Source: CAD feature listing. Evaluate the final solid. Frame: model axes, mm. Coordinates: 2 decimals unless noted, no trailing zeros. Loops run counter-clockwise (first coordinate to the right, second up) from the corner with the lowest first, then second, coordinate; pieces in that order, holes last. Notation, with made-up numbers: (70, 5) -> (105, 5) arc R19 ccw to (105, 27) -> close; hole circle Ø8 at (44.5, 63). An arc over 180 degrees is marked (long way). Answer as a JSON object with one key per item and string values. Group by question number.
from build123d import *

# Parameters (mm, degrees)
F0_W         = 150
F0_H         = 73.4827055006
F0_R         = 15.3666463422
F0_R_2       = 9.9309311283
F1_DEPTH     = 76.962
F2_T1_DEPTH  = 139.84
F2_T3_DEPTH  = 63.3227055006
F2_T5_DEPTH  = 157.62
F2_T7_DEPTH  = 81.1027055006
F2_T9_DEPTH  = 84.582
F2_S13_W     = 5.08
F2_S13_H     = 5.08
F2_T14_DEPTH = 5.08
F2_S19_W     = 5.08
F2_S19_H     = 5.08
F2_T20_DEPTH = 5.08
F2_S25_W     = 5.08
F2_S25_H     = 5.08
F2_T26_DEPTH = 5.08


# Not quite as in the source:
# - a fillet or chamfer that OpenCascade refuses, or shapes differently, is made with other operations: its cross-section is extruded or revolved along the edge and cut away or added


with BuildPart() as f1:
    # F0 (on Top) → F1 (new body)
    with BuildSketch(Plane.XY):
        with Locations((19.2005559802, -34.1252638027)):
            Rectangle(F0_W, F0_H)
        with Locations((51.502276212, -42.9059304297)):
            Circle(F0_R, mode=Mode.SUBTRACT)
        with Locations((-28.6887511611, -14.8067288101)):
            Circle(F0_R_2, mode=Mode.SUBTRACT)
    extrude(amount=F1_DEPTH)

    # F2: fillet of radius 5.08 on 9 edges, made by hand

    # F2_s2 → F2_t1 (cut)
    with BuildSketch(Plane.YZ.offset(-50.7194440198)):
        with BuildLine():
            ThreePointArc((-70.866616553, 71.882), (-69.3787190014, 75.4741024484), (-65.786616553, 76.962))
            Line((-65.786616553, 76.962), (-70.866616553, 76.962))
            Line((-70.866616553, 76.962), (-70.866616553, 71.882))
        make_face()
    extrude(amount=F2_T1_DEPTH, mode=Mode.SUBTRACT)

    # F2_s4 → F2_t3 (cut)
    with BuildSketch(Plane.XZ.offset(2.4639110524)):
        with BuildLine():
            ThreePointArc((94.2005559802, 71.882), (92.7126584286, 75.4741024484), (89.1205559802, 76.962))
            Line((89.1205559802, 76.962), (94.2005559802, 76.962))
            Line((94.2005559802, 76.962), (94.2005559802, 71.882))
        make_face()
    extrude(amount=F2_T3_DEPTH, mode=Mode.SUBTRACT)

    # F2_s6 → F2_t5 (cut)
    with BuildSketch(Plane.YZ.offset(-68.4994440198)):
        with BuildLine():
            ThreePointArc((2.6160889476, 71.882), (1.128191396, 75.4741024484), (-2.4639110524, 76.962))
            Line((-2.4639110524, 76.962), (2.6160889476, 76.962))
            Line((2.6160889476, 76.962), (2.6160889476, 71.882))
        make_face()
    extrude(amount=F2_T5_DEPTH, mode=Mode.SUBTRACT)

    # F2_s8 → F2_t7 (cut)
    with BuildSketch(Plane.XZ.offset(-15.3160889476)):
        with BuildLine():
            ThreePointArc((-55.7994440198, 71.882), (-54.3115464682, 75.4741024484), (-50.7194440198, 76.962))
            Line((-50.7194440198, 76.962), (-55.7994440198, 76.962))
            Line((-55.7994440198, 76.962), (-55.7994440198, 71.882))
        make_face()
    extrude(amount=F2_T7_DEPTH, mode=Mode.SUBTRACT)

    # F2_s10 → F2_t9 (cut)
    with BuildSketch(Plane.XY.offset(-12.7)):
        with BuildLine():
            ThreePointArc((89.1205559802, -70.866616553), (92.7126584286, -69.3787190014), (94.2005559802, -65.786616553))
            Line((94.2005559802, -65.786616553), (94.2005559802, -70.866616553))
            Line((94.2005559802, -70.866616553), (89.1205559802, -70.866616553))
        make_face()
        with BuildLine():
            ThreePointArc((89.1205559802, 2.6160889476), (92.7126584286, 1.128191396), (94.2005559802, -2.4639110524))
            Line((94.2005559802, -2.4639110524), (94.2005559802, 2.6160889476))
            Line((94.2005559802, 2.6160889476), (89.1205559802, 2.6160889476))
        make_face()
        with BuildLine():
            ThreePointArc((-55.7994440198, -65.786616553), (-54.3115464682, -69.3787190014), (-50.7194440198, -70.866616553))
            Line((-50.7194440198, -70.866616553), (-55.7994440198, -70.866616553))
            Line((-55.7994440198, -70.866616553), (-55.7994440198, -65.786616553))
        make_face()
    extrude(amount=F2_T9_DEPTH, mode=Mode.SUBTRACT)


with BuildPart() as f2_tool12:
    # F2_s13 → F2_t14 (new body)
    with BuildSketch(Plane.YZ.offset(-50.7194440198)):
        with Locations((-68.326616553, 74.422)):
            Rectangle(F2_S13_W, F2_S13_H)
    extrude(amount=-F2_T14_DEPTH)

    # F2_s15 → F2_t16 (revolve, cut)
    with BuildSketch(Plane(origin=(-50.7194440198, -65.786616553, 71.882), x_dir=(0, 0.7071067812, -0.7071067812), z_dir=(0, 0.7071067812, 0.7071067812))):
        with BuildLine():
            ThreePointArc((0, -5.08), (5.08, 0), (0, 5.08))
            Line((0, 5.08), (0, -5.08))
        make_face()
    revolve(axis=Axis((-50.7194440198, -65.786616553, 71.882), (-1, 0, 0)), mode=Mode.SUBTRACT)


with BuildPart() as f1_1:
    add(f1.part)

    # F2_t11: cut F2_tool12
    add(f2_tool12.part, mode=Mode.SUBTRACT)


with BuildPart() as f2_tool18:
    # F2_s19 → F2_t20 (new body)
    with BuildSketch(Plane.XZ.offset(65.786616553)):
        with Locations((91.6605559802, 74.422)):
            Rectangle(F2_S19_W, F2_S19_H)
    extrude(amount=F2_T20_DEPTH)

    # F2_s21 → F2_t22 (revolve, cut)
    with BuildSketch(Plane(origin=(89.1205559802, -65.786616553, 71.882), x_dir=(-0.7071067812, 0, -0.7071067812), z_dir=(-0.7071067812, 0, 0.7071067812))):
        with BuildLine():
            ThreePointArc((0, -5.08), (5.08, 0), (0, 5.08))
            Line((0, 5.08), (0, -5.08))
        make_face()
    revolve(axis=Axis((89.1205559802, -65.786616553, 71.882), (0, -1, 0)), mode=Mode.SUBTRACT)


with BuildPart() as f1_2:
    add(f1_1.part)

    # F2_t17: cut F2_tool18
    add(f2_tool18.part, mode=Mode.SUBTRACT)


with BuildPart() as f2_tool24:
    # F2_s25 → F2_t26 (new body)
    with BuildSketch(Plane.XZ.offset(2.4639110524)):
        with Locations((91.6605559802, 74.422)):
            Rectangle(F2_S25_W, F2_S25_H)
    extrude(amount=-F2_T26_DEPTH)

    # F2_s27 → F2_t28 (revolve, cut)
    with BuildSketch(Plane(origin=(89.1205559802, -2.4639110524, 71.882), x_dir=(-0.7071067812, 0, -0.7071067812), z_dir=(0.7071067812, 0, -0.7071067812))):
        with BuildLine():
            ThreePointArc((0, -5.08), (5.08, 0), (0, 5.08))
            Line((0, 5.08), (0, -5.08))
        make_face()
    revolve(axis=Axis((89.1205559802, -2.4639110524, 71.882), (0, 1, 0)), mode=Mode.SUBTRACT)


with BuildPart() as f1_3:
    add(f1_2.part)

    # F2_t23: cut F2_tool24
    add(f2_tool24.part, mode=Mode.SUBTRACT)

    # F2_s29 → F2_t30 (revolve, cut)
    with BuildSketch(Plane.XZ.offset(42.9059304297)):
        with BuildLine():
            ThreePointArc((66.8689225542, 71.882), (68.3568201058, 75.4741024484), (71.9489225542, 76.962))
            Line((71.9489225542, 76.962), (66.8689225542, 76.962))
            Line((66.8689225542, 76.962), (66.8689225542, 71.882))
        make_face()
    revolve(axis=Axis((51.502276212, -42.9059304297, 76.962), (0, 0, 1)), mode=Mode.SUBTRACT)

    # F2_s31 → F2_t32 (revolve, cut)
    with BuildSketch(Plane.XZ.offset(14.8067288101)):
        with BuildLine():
            ThreePointArc((-18.7578200328, 71.882), (-17.2699224813, 75.4741024484), (-13.6778200328, 76.962))
            Line((-13.6778200328, 76.962), (-18.7578200328, 76.962))
            Line((-18.7578200328, 76.962), (-18.7578200328, 71.882))
        make_face()
    revolve(axis=Axis((-28.6887511611, -14.8067288101, 76.962), (0, 0, 1)), mode=Mode.SUBTRACT)


solid = f1_3.part
1. Pin query (flat end, axial travel): pin 1 Ø18.5 at (x, y) = (51.5, -42.91) entering from +Z. Return the tip coordinate at first contact, or that it passes through.
2. Ray query, L1, parallel to X at y = -15, z = 56.5; L2, parallel to X at y = -31, z = 3; L3, parallel to Y at x = 48, z = 67. Return the intervals inside material, ascending.
3. Section query A-A on z = 8.5. Return loops of the section in (x, y).
Solved:
{
 "1": {"pin 1": "through"},
 "2": {"L1": "-55.8 to -38.62, -18.76 to 94.2", "L2": "-55.8 to 41.79, 61.22 to 94.2", "L3": "-70.87 to -57.87, -27.94 to 2.62"},
 "3": {"outline": "(-55.8, -65.79) arc R5.08 ccw to (-50.72, -70.87) -> (89.12, -70.87) arc R5.08 ccw to (94.2, -65.79) -> (94.2, -2.46) arc R5.08 ccw to (89.12, 2.62) -> (-55.8, 2.62) -> close; hole circle Ø19.86 at (-28.69, -14.81); hole circle Ø30.73 at (51.5, -42.91)"}
}
